```python
from build123d import *

# Parameters (mm, degrees)
SKETCH062_W             = 372
SKETCH062_H             = 88
PAD023_DEPTH            = 12
SKETCH063_W             = 8
SKETCH063_H             = 88
POCKET038_DEPTH         = 8
SKETCH064_W             = 364
SKETCH064_H             = 6
POCKET039_DEPTH         = 6
BODY022_ROLL_ANGLE      = 90
BODY022_PLACEMENT_ANGLE = -90


with BuildPart() as part:
    # Sketch062 → Pad023 (new body)
    with BuildSketch(Plane.XY):
        with Locations((0, 44)):
            Rectangle(SKETCH062_W, SKETCH062_H)
    extrude(amount=PAD023_DEPTH)

    # Sketch063 (on Face5 of Pad023) → Pocket038 (cut)
    with BuildSketch(Plane(origin=(0, 0, 0), x_dir=(1, 0, 0), z_dir=(0, 0, -1))):
        with Locations((-182, -44)):
            Rectangle(SKETCH063_W, SKETCH063_H)
    pocket038 = extrude(amount=-POCKET038_DEPTH, mode=Mode.SUBTRACT)

    # Mirrored014: Pocket038 across Sketch063 V_Axis
    add(pocket038.mirror(Plane(origin=(0, 0, 0), x_dir=(0, 0, -1), z_dir=(1, 0, 0))), mode=Mode.SUBTRACT)

    # Sketch064 (on Face3 of Mirrored014) → Pocket039 (cut)
    with BuildSketch(Plane(origin=(0, 0, 0), x_dir=(1, 0, 0), z_dir=(0, 0, -1))):
        with Locations((0, -9)):
            Rectangle(SKETCH064_W, SKETCH064_H)
    extrude(amount=-POCKET039_DEPTH, mode=Mode.SUBTRACT)


with BuildPart() as part_1:
    # Body022 roll: moved
    add(part.part.rotate(Axis((0, 0, 0), (1, 0, 0)), BODY022_ROLL_ANGLE))


with BuildPart() as part_2:
    # Body022 placement: moved
    add(part_1.part.moved(Location((-220.3, 178, 0))).rotate(Axis((-220.3, 178, 0), (0, 0, 1)), BODY022_PLACEMENT_ANGLE))


solid = part_2.part
```
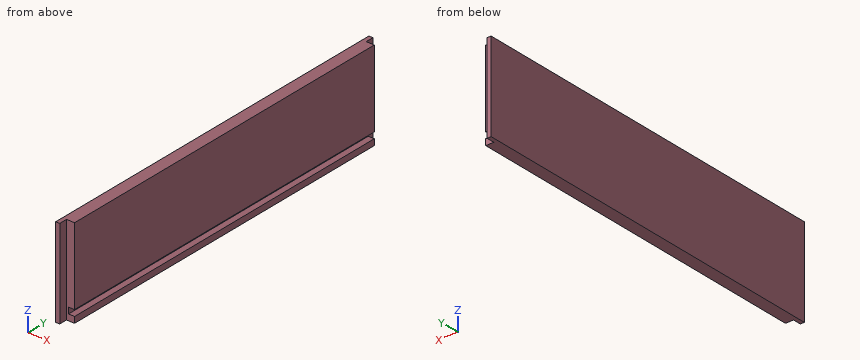
Could you check a few things on this model? Use its own coordinates, in mm. Round coordinates to 2 decimals unless told otherwise and drop trailing zeros. Loops run counter-clockwise (first coordinate to the right, second up) from the corner with the lowest first, then second, coordinate; pieces in that order, holes last. Notation, with made-up numbers: M 39.25,85.25 L 72.25,85.25 A13 ccw 72.25,96.25 Z; hole C -29,-33.75 d5. An arc over 180 degrees is marked long. Answer as CSV lines item,"result".
1) Imagine slicing it at A-A on x = -223.75. List the corners of the cut face in (y, z) for me, and give its area (3 significant figures).
From the geometry:
outline,"M 0,0 L 356,0 L 356,6 L 0,6 Z; M 0,12 L 356,12 L 356,88 L 0,88 Z"
area,"29,200 mm^2"
2) Imagine slicing it at C-C on y = 245. List the corners of the cut face in (x, z) for me, and give its area (3 significant figures).
From the geometry:
outline,"M -232.3,0 L -220.3,0 L -220.3,6 L -226.3,6 L -226.3,12 L -220.3,12 L -220.3,88 L -232.3,88 Z"
area,"1,020 mm^2"
3) For pin 1 Ø2.5 at (y, z) = (358.5, 60.5) entering from +X; pin 2 Ø4 at (x, z) = (-224, 52) entering from +Y; pin 3 Ø1 at (x, z) = (-227.5, 54) entering from -Y, each with a flat end and sliding along its axis, tell me the tip position at first contact or that it passes through.
From the geometry:
pin 1,"x = -228.3"
pin 2,"y = 356"
pin 3,"y = 0"
4) Imagine slicing it at B-B on z = 37. List the corners of the cut face in (x, y) for me, and give its area (3 significant figures).
From the geometry:
outline,"M -232.3,-8 L -228.3,-8 L -228.3,0 L -220.3,0 L -220.3,356 L -228.3,356 L -228.3,364 L -232.3,364 Z"
area,"4,340 mm^2"
5) If I drill on probe 1 along Z at (x, y) = (-222.75, 76); probe 2 along X at (y, z) = (49.5, 10); probe 3 along Y at (x, z) = (-227.5, 78.5), over which ranges is the centre line in solid material (lowest first)?
From the geometry:
probe 1,"0 to 6, 12 to 88"
probe 2,"-232.3 to -226.3"
probe 3,"0 to 356"
